from build123d import *

# Parameters (mm, degrees)
SKETCH2_W           = 42
SKETCH2_H           = 8
BOSS_EXTRUDE1_DEPTH = 23
SKETCH3_W           = 42
SKETCH3_H           = 8
BOSS_EXTRUDE2_DEPTH = 74
CUT_EXTRUDE1_DEPTH  = 100.659420026
BOSS_EXTRUDE3_DEPTH = 5
BOSS_EXTRUDE5_DEPTH = 5
SKETCH11_R          = 7
CUT_EXTRUDE2_DEPTH  = 100.659420026


with BuildPart() as part:
    # Sketch2 → Boss-Extrude1 (new, symmetric)
    with BuildSketch(Plane.XY):
        with Locations((21, 4)):
            Rectangle(SKETCH2_W, SKETCH2_H)
    extrude(amount=BOSS_EXTRUDE1_DEPTH, both=True)

    # Sketch3 → Boss-Extrude2 (add)
    with BuildSketch(Plane(origin=(0, 8, 0), x_dir=(1, 0, 0), z_dir=(0, 1, 0))):
        with Locations((21, 19)):
            Rectangle(SKETCH3_W, SKETCH3_H)
    extrude(amount=BOSS_EXTRUDE2_DEPTH)

    # Sketch4 → Cut-Extrude1 (cut, through all)
    with BuildSketch(Plane.XY.offset(-15)):
        Polygon((0, 82), (12, 82), (0, 62), align=None)
        Polygon((30, 82), (42, 82), (42, 62), align=None)
    extrude(amount=-CUT_EXTRUDE1_DEPTH, mode=Mode.SUBTRACT)

    # Sketch6 → Boss-Extrude3 (add)
    with BuildSketch(Plane(origin=(0, 0, 0), x_dir=(0, 0, -1), z_dir=(1, 0, 0))):
        Polygon((15, 45), (-15, 8), (15, 8), align=None)
    extrude(amount=BOSS_EXTRUDE3_DEPTH)

    # Sketch10 → Boss-Extrude5 (add)
    with BuildSketch(Plane(origin=(42, 0, 0), x_dir=(0, 0, -1), z_dir=(1, 0, 0))):
        Polygon((15, 45), (-15, 8), (15, 8), align=None)
    extrude(amount=-BOSS_EXTRUDE5_DEPTH)

    # Sketch11 → Cut-Extrude2 (cut, through all)
    with BuildSketch(Plane.XY.offset(-15)):
        with Locations((21, 62)):
            Circle(SKETCH11_R)
    extrude(amount=-CUT_EXTRUDE2_DEPTH, mode=Mode.SUBTRACT)


solid = part.part
The listing builds one solid part. Answer for the finished solid, in the listing's coordinates (mm). A direction names the side the tool comes from. Round coordinates to 2 decimals unless told otherwise and drop trailing zeros. Write each loop counter-clockwise with the first axis right and the second up, starting at its lowest first coordinate (ties: lowest second). Pieces come first, ordered by that corner, then holes. Notation, with made-up numbers: M 38.5,-34.75 L 49.5,-34.75 A18 cw 49.5,-0.75 Z; hole C -40,80.5 d7. An arc over 180 degrees is marked long. Write each question's results on one line, items separated by ' | '. Start each with the question number.
Item 1: For faces 5 (the face through (37, 19, -6)), 6 (the face through (0, 25, -10)), determine the directions among +Z, -Z, +X, -X, +Y, -Y from which every point of the face is accessible in a straight line to the end or side of a thin tool.
Item 2: A cutting plane is placed at D-D on y = 42. Write down the section's boundary in (x, z), and give its area (3 significant figures).
Item 3: Flat-ended cylindrical pins translate along their axes: pin 1 Ø6 at (x, z) = (29, -12.5) entering from +Y; pin 2 Ø6 at (x, z) = (14, 4) entering from +Y; pin 3 Ø1.5 at (x, y) = (27.5, 10.5) entering from +Z; pin 4 Ø10 at (y, z) = (39.5, -2) entering from +X. Find the tip coordinate at first contact, or state that the pin passes through.
Item 4: A cutting plane is placed at B-B on x = 22. Write down the section's boundary in (y, z).
Item 5: For a pull along X with two mould halves and no side action, classify faces 1 (the face through (21, 44, -15)), 2 (the face through (21, 82, -19)), 3 (the face through (42, 25, -10)), 4 (the face through (5, 19, -6)) as pulls with the +X half, pulls with the -X half, needs draft (parallel to the pull), parting line crosses it, or undercut.
Item 6: A cutting plane is placed at A-A on z = -17. Write down the section's boundary in (x, y).
Item 7: Straight lines are drawn through the part: L1, parallel to X at y = 27.5, z = -14; L2, parallel to Y at x = 21, z = -18; L3, parallel to Z at x = 13.5, y = 44. For each, find the intervals that lie inside material, in ascending order. Write a range as [from, to].
Item 8: A cutting plane is placed at C-C on z = 10. Write down the section's boundary in (x, y), and give its area (3 significant figures).
Check sheet entries:
1) face 5: +Z, +Y | face 6: +Z, -Z, -X, +Y, -Y
2) outline: M 0,-23 L 42,-23 L 42,-12.57 L 37,-12.57 L 37,-15 L 5,-15 L 5,-12.57 L 0,-12.57 Z | area: 360 mm²
3) pin 1: y = 82 | pin 2: y = 8 | pin 3: z = -15 | pin 4: through
4) outline: M 0,-23 L 55.07,-23 L 55.07,-15 L 8,-15 L 8,23 L 0,23 Z; M 68.93,-23 L 82,-23 L 82,-15 L 68.93,-15 Z
5) face 1: undercut | face 2: needs draft | face 3: pulls with the +X half | face 4: undercut
6) outline: M 0,0 L 42,0 L 42,62 L 30,82 L 12,82 L 0,62 Z; hole C 21,62 d14
7) L1: [0, 5], [37, 42] | L2: [0, 55], [69, 82] | L3: [-23, -15]
8) outline: M 0,0 L 42,0 L 42,14.17 L 37,14.17 L 37,8 L 5,8 L 5,14.17 L 0,14.17 Z | area: 398 mm²
